from build123d import *

# Parameters (mm, degrees)
F0_R     = 1.5
F0_R_2   = 11
F0_R_3   = 3
F1_DEPTH = 2
F2_SIZE  = 5


with BuildPart() as f1:
    # F0 (on Top) → F1 (new body)
    with BuildSketch(Plane.XY):
        Polygon((-36, -37.666667), (36, -37.666667), (36, 4.333333), (6, 4.333333), (6, 34.333333), (-36, 34.333333), align=None)
        with Locations((-30.5, -32.166667)):
            Circle(F0_R, mode=Mode.SUBTRACT)
        with Locations((-15, -16.666667)):
            Circle(F0_R_2, mode=Mode.SUBTRACT)
        with Locations((0.5, -32.166667)):
            Circle(F0_R, mode=Mode.SUBTRACT)
        with Locations((21, -16.666667)):
            Circle(F0_R_3, mode=Mode.SUBTRACT)
        with Locations((-30.5, -1.166667)):
            Circle(F0_R, mode=Mode.SUBTRACT)
        with Locations((-15, 19.333333)):
            Circle(F0_R_3, mode=Mode.SUBTRACT)
        with Locations((0.5, -1.166667)):
            Circle(F0_R, mode=Mode.SUBTRACT)
    extrude(amount=F1_DEPTH)

    # F2
    f2_edges = [f1.edges().sort_by_distance(p)[0] for p in [
        (-36, -37.666667, 1),
    ]]
    chamfer(f2_edges, length=F2_SIZE)


solid = f1.part
Could you check a few things on this model? Use its own coordinates, in mm. Give positions to 0.01 mm unless a question says otherwise; leave off trailing zeros. Write each loop counter-clockwise with the first axis right and the second up, starting at its lowest first coordinate (ties: lowest second). Pieces come first, ordered by that corner, then holes. Notation, with made-up numbers: (23.25, 63.5) - (75.25, 63.5) arc R22 ccw to (75.25, 97.5) - close; hole circle Ø8 at (-32, 42.5). An arc over 180 degrees is marked (long way). Use CSV: the item, a comma, the result in double quotes. Start each with the question number.
Item 1: If we mould it in two halves opening along Y, with no side actions, what happens to faces 1 (the face through (6, 19, 1)), 2 (the face through (18.79, -14.64, 0.99)), 3 (the face through (-4.84, -20.88, 0.99)), 4 (the face through (21, 4.333, 1))? For each: pulls with the +Y half, pulls with the -Y half, needs draft (parallel to the pull), parting line crosses it, or undercut.
Item 2: I want a section at A-A, the plane x = 21. Please give me the cut outline in (y, z).
Item 3: If I drill on line 1 along Y through (x, z) = (0.5, 1.3); line 2 along Y through (x, z) = (-15, 0.7); line 3 along X through (y, z) = (-17, 0.5), over which ranges is the centre line in solid material (lowest first)?
Item 4: I want a section at B-B, the plane x = 0.5. Please give me the cut outline in (y, z).
Item 5: I'm going to push flat-ended pins straight in: pin 1 (2.5 mm diameter, centred on x = 0.5, y = -1.17, fed in from -Z); pin 2 (1 mm diameter, centred on x = 27.5, z = 1, fed in from +Y). Where does each tip first touch, or does it pass through?
Item 6: I want a section at D-D, the plane z = 1.2. Please give me the cut outline in (x, y).
Item 7: I want a section at C-C, the plane y = -25. Please give me the cut outline in (x, z).
Findings:
1,face 1,"needs draft"
1,face 2,"undercut"
1,face 3,"undercut"
1,face 4,"pulls with the +Y half"
2,outline,"(-37.67, 0) - (-19.67, 0) - (-19.67, 2) - (-37.67, 2) - close; (-13.67, 0) - (4.33, 0) - (4.33, 2) - (-13.67, 2) - close"
3,line 1,"y = -37.67 to -33.67, -30.67 to -2.67, 0.33 to 34.33"
3,line 2,"y = -37.67 to -27.67, -5.67 to 16.33, 22.33 to 34.33"
3,line 3,"x = -36 to -25.99, -4.01 to 18.02, 23.98 to 36"
4,outline,"(-37.67, 0) - (-33.67, 0) - (-33.67, 2) - (-37.67, 2) - close; (-30.67, 0) - (-2.67, 0) - (-2.67, 2) - (-30.67, 2) - close; (0.33, 0) - (34.33, 0) - (34.33, 2) - (0.33, 2) - close"
5,pin 1,"passes through"
5,pin 2,"stops at y = 4.33"
6,outline,"(-36, -32.67) - (-31, -37.67) - (36, -37.67) - (36, 4.33) - (6, 4.33) - (6, 34.33) - (-36, 34.33) - close; hole circle Ø3 at (-30.5, -32.17); hole circle Ø3 at (-30.5, -1.17); hole circle Ø22 at (-15, -16.67); hole circle Ø6 at (-15, 19.33); hole circle Ø3 at (0.5, -32.17); hole circle Ø3 at (0.5, -1.17); hole circle Ø6 at (21, -16.67)"
7,outline,"(-36, 0) - (-22.18, 0) - (-22.18, 2) - (-36, 2) - close; (-7.82, 0) - (36, 0) - (36, 2) - (-7.82, 2) - close"
